Part model, mm, in its own coordinate system. Face numbers are marked on the shaded views. A direction names the side the tool comes from. Coordinates: 2 decimals unless noted, no trailing zeros. Order: outer loops, then holes, each group sorted by start corner. A loop starts at its lowest first (then second) coordinate and runs counter-clockwise, first axis right, second up.
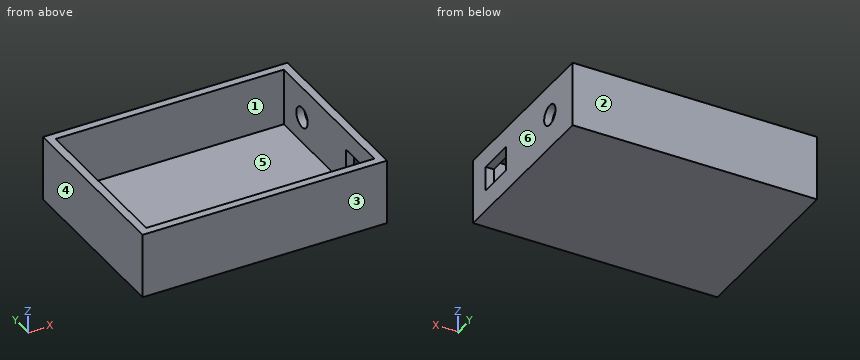
```python
from build123d import *

# Parameters (mm, degrees)
F0_W     = 95.25
F0_H     = 69.85
F0_W_2   = 88.9
F0_H_2   = 63.5
F1_DEPTH = 25.4
F3_DEPTH = 3.175
F5_D     = 7.9375
F5_DEPTH = 12.7
F2_W     = 14.2875
F2_H     = 9.525
F6_DEPTH = 12.7


with BuildPart() as f1:
    # F0 (on Top) → F1 (new body)
    with BuildSketch(Plane.XY):
        Rectangle(F0_W, F0_H)
        Rectangle(F0_W_2, F0_H_2, mode=Mode.SUBTRACT)
    extrude(amount=F1_DEPTH)

    # F0 (on Top) → F3 (join)
    with BuildSketch(Plane.XY):
        Rectangle(F0_W_2, F0_H_2)
    extrude(amount=F3_DEPTH)

    # F5
    with Locations(Plane.YZ.offset(47.625)):
        with Locations((18.973511, 13.251342)):
            Hole(F5_D / 2, depth=F5_DEPTH)

    # F2 (on face) → F6 (cut, symmetric)
    with BuildSketch(Plane.YZ.offset(47.625)):
        with Locations((-18.882488, 13.021725)):
            Rectangle(F2_W, F2_H)
    extrude(amount=F6_DEPTH, both=True, mode=Mode.SUBTRACT)


solid = f1.part
```
(1) Probe line 1 (X direction, y = -9, z = 11.75) (3 decimals); line 2 (Y direction, x = 13, z = 17) (3 decimals); line 3 (Z direction, x = 0, y = 21.5) (3 decimals). List the from-to ranges inside material, lowest first.
(2) Slice it at C-C, the plane x = -3. Give the cut face in (y, z) (3 decimals), then the cut area to 3 significant figures.
(3) Slice it at A-A, the plane y = -25. Give the cut face in (x, z) (3 decimals), then the cut area to 3 significant figures.
(4) Drop flat-ended pins along their axis: pin 1 (1.5 mm diameter, centred on x = -9, y = 17.5, fed in from +Z) (3 decimals); pin 2 (7 mm diameter, centred on y = 18.97, z = 13.25, fed in from +X); pin 3 (4 mm diameter, centred on x = -8, y = -8, fed in from -Z). Give the stop position or say it passes through.
(5) Slice it at B-B, the plane z = 7. Give the cut face in (x, y) (3 decimals), then the cut area to 3 significant figures.
(6) Tool access for the marked faces 1 and 2: list every direction of +Z, -Z, +X, -X, +Y, -Y with a clear straight run to the whole face (end or side of a thin tool).
(7) Pull direction X, two halves, no side cores. Call the marked faces 3, 4, 5 and 6: +X half, -X half, draft (parallel to the pull), parting line (faces both ways), or undercut.
(8) Slice it at D-D, the plane y = -6. Give the cut face in (x, z) (3 decimals).
Here are the results:
1. line 1: x = -47.625 to -44.45, 44.45 to 47.625
1. line 2: y = -34.925 to -31.75, 31.75 to 34.925
1. line 3: z = 0 to 3.175
2. outline: (-34.925, 0) - (34.925, 0) - (34.925, 25.4) - (31.75, 25.4) - (31.75, 3.175) - (-31.75, 3.175) - (-31.75, 25.4) - (-34.925, 25.4) - close
2. area: 363 mm2
3. outline: (-47.625, 0) - (47.625, 0) - (47.625, 8.259) - (44.45, 8.259) - (44.45, 3.175) - (-44.45, 3.175) - (-44.45, 25.4) - (-47.625, 25.4) - close; (44.45, 17.784) - (47.625, 17.784) - (47.625, 25.4) - (44.45, 25.4) - close
3. area: 413 mm2
4. pin 1: stops at z = 3.175
4. pin 2: stops at x = -44.45
4. pin 3: stops at z = 0
5. outline: (-47.625, -34.925) - (47.625, -34.925) - (47.625, 34.925) - (-47.625, 34.925) - close; hole (-44.45, -31.75) - (44.45, -31.75) - (44.45, 31.75) - (-44.45, 31.75) - close
5. area: 1,010 mm2
6. face 1: +Z
6. face 2: +Z, -Z, +X, -X, +Y
7. face 3: draft
7. face 4: -X half
7. face 5: undercut
7. face 6: +X half
8. outline: (-47.625, 0) - (47.625, 0) - (47.625, 25.4) - (44.45, 25.4) - (44.45, 3.175) - (-44.45, 3.175) - (-44.45, 25.4) - (-47.625, 25.4) - close
